from build123d import *

# Parameters (mm, degrees)
F0_W     = 120
F0_H     = 120
F0_W_2   = 100
F0_H_2   = 100
F1_DEPTH = 22
F2_R     = 7.5
F3_DEPTH = 237
F4_R     = 7.5
F5_DEPTH = 185


with BuildPart() as f1:
    # F0 (on Top) → F1 (new body)
    with BuildSketch(Plane.XY):
        with Locations((56.498835, 49.731983)):
            Rectangle(F0_W, F0_H)
        with Locations((56.498835, 49.731983)):
            Rectangle(F0_W_2, F0_H_2, mode=Mode.SUBTRACT)
    extrude(amount=F1_DEPTH)

    # F2 (on face) → F3 (cut)
    with BuildSketch(Plane.XZ.offset(10.268017)):
        with Locations((56.498835, 11)):
            Circle(F2_R)
    extrude(amount=-F3_DEPTH, mode=Mode.SUBTRACT)

    # F4 (on face) → F5 (cut)
    with BuildSketch(Plane(origin=(-3.501165, 0, 0), x_dir=(0, -1, 0), z_dir=(-1, 0, 0))):
        with Locations((-49.731983, 11)):
            Circle(F4_R)
    extrude(amount=-F5_DEPTH, mode=Mode.SUBTRACT)


solid = f1.part
The model under review builds one solid part; all positions refer to its coordinate system, in mm. A direction names the side the tool comes from. Round coordinates to 2 decimals unless told otherwise and drop trailing zeros. Loops run counter-clockwise (first coordinate to the right, second up) from the corner with the lowest first, then second, coordinate; pieces in that order, holes last. Notation, with made-up numbers: M 49.25,14.25 L 56.25,14.25 A21 ccw 56.25,42.25 Z; hole C -19.75,54 d11. An arc over 180 degrees is marked long. Answer as a JSON object with one key per item and string values.
Item 1: Clearance check with a flat-ended pin moving along its axis: P1, Ø12, axis at x = 56.5, z = 11, coming from the -Y side. State where the tip first meets the part, or that it passes through.
Check sheet entries:
{"P1": "through"}
Item 2: The part is to be moulded in two halves that separate along X. For faces 3 (the face through (63.652, -5.338, 13.253)), 4 (the face through (1.429, 46.271, 4.346)), 5 (the face through (-3.501, 49, 1)), say which applies: +X half, -X half, draft (parallel to the pull), parting line (faces both ways), or undercut.
Check sheet entries:
{"face 3": "undercut", "face 4": "draft", "face 5": "-X half"}
Item 3: We need section B-B, the plane z = 11. State the section outline as (x, y) points.
Check sheet entries:
{"outline": "M -3.5,-10.27 L 49,-10.27 L 49,-0.27 L 6.5,-0.27 L 6.5,42.23 L -3.5,42.23 Z; M -3.5,57.23 L 6.5,57.23 L 6.5,99.73 L 49,99.73 L 49,109.73 L -3.5,109.73 Z; M 64,-10.27 L 116.5,-10.27 L 116.5,42.23 L 106.5,42.23 L 106.5,-0.27 L 64,-0.27 Z; M 64,99.73 L 106.5,99.73 L 106.5,57.23 L 116.5,57.23 L 116.5,109.73 L 64,109.73 Z"}
Item 4: For line 1 along X through (y, z) = (25.5, 12.75); line 2 along Y through (x, z) = (63, 1.75); line 3 along X through (y, z) = (-1, 12.25), list the stretches that pass through material, from the lowest coordinate up.
Check sheet entries:
{"line 1": "-3.5 to 6.5, 106.5 to 116.5", "line 2": "-10.27 to -0.27, 99.73 to 109.73", "line 3": "-3.5 to 49.1, 63.89 to 116.5"}
Item 5: We need section D-D, the plane x = 84.5. State the section outline as (y, z) points, and give its area (3 significant figures).
Check sheet entries:
{"outline": "M -10.27,0 L -0.27,0 L -0.27,22 L -10.27,22 Z; M 99.73,0 L 109.73,0 L 109.73,22 L 99.73,22 Z", "area": "440 mm2"}
Item 6: Tool access review of faces 1 (the face through (56, 109.732, 1)), 2 (the face through (106.499, 49, 1)): name each direction out of +Z, -Z, +X, -X, +Y, -Y from which nothing blocks a thin tool from reaching the whole face with its end or side.
Check sheet entries:
{"face 1": "+Z, -Z, +X, -X, +Y", "face 2": "+Z, -Z"}
Item 7: We need section A-A, the plane x = 56.5. State the section outline as (y, z) points.
Check sheet entries:
{"outline": "M -10.27,0 L -0.27,0 L -0.27,3.5 L -10.27,3.5 Z; M -10.27,18.5 L -0.27,18.5 L -0.27,22 L -10.27,22 Z; M 99.73,0 L 109.73,0 L 109.73,3.5 L 99.73,3.5 Z; M 99.73,18.5 L 109.73,18.5 L 109.73,22 L 99.73,22 Z"}
Item 8: We need section C-C, the plane y = 81.5. State the section outline as (x, z) points, and give its area (3 significant figures).
Check sheet entries:
{"outline": "M -3.5,0 L 6.5,0 L 6.5,22 L -3.5,22 Z; M 106.5,0 L 116.5,0 L 116.5,22 L 106.5,22 Z", "area": "440 mm2"}
